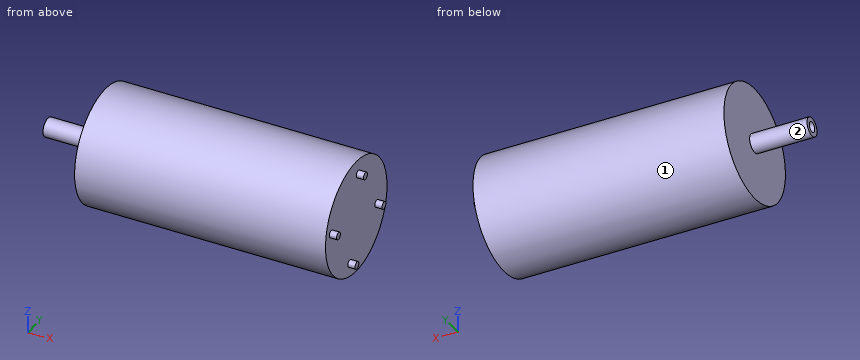
```python
from build123d import *

# Parameters (mm, degrees)
F0_W     = 40
F0_H     = 3
F2_R     = 2.5
F3_DEPTH = 5


with BuildPart() as f1:
    # F0 (on Front) → F1 (revolve)
    with BuildSketch(Plane.XZ):
        with Locations((-34.818123, 5)):
            Rectangle(F0_W, F0_H)
        Polygon((-14.818123, 3.5), (-14.818123, 0), (160.181877, 0), (160.181877, 40), (-14.818123, 40), (-14.818123, 6.5), align=None)
    revolve(axis=Axis((18.749876, 0, 0), (1, 0, 0)))

    # F2 (on face) → F3 (join)
    with BuildSketch(Plane.YZ.offset(160.181877)):
        with Locations((2.648871, 29.522968)):
            Circle(F2_R)
        with Locations((-8.448871, -29.522968)):
            Circle(F2_R)
        with Locations((26.622968, -5.548871)):
            Circle(F2_R)
        with Locations((-32.422968, 5.548871)):
            Circle(F2_R)
    extrude(amount=F3_DEPTH)


solid = f1.part
```
Work out the finished part from the listing and answer in its coordinate system (mm). Face numbers are marked on the shaded views. A direction names the side the tool comes from. Give positions to 0.01 mm unless a question says otherwise; leave off trailing zeros. Order: outer loops, then holes, each group sorted by start corner. A loop starts at its lowest first (then second) coordinate and runs counter-clockwise, first axis right, second up.
1. Section D-D, the plane z = -20 is taken. Determine the outline of the cut face in (x, y).
Result sheet:
outline: (-14.82, -34.64) - (160.18, -34.64) - (160.18, 34.64) - (-14.82, 34.64) - close
2. Section A-A, the plane z = 0 is taken. Determine the outline of the cut face in (x, y), and give its area (3 significant figures).
Result sheet:
outline: (-54.82, -6.5) - (-14.82, -6.5) - (-14.82, -40) - (160.18, -40) - (160.18, 40) - (-14.82, 40) - (-14.82, 6.5) - (-54.82, 6.5) - (-54.82, 3.5) - (-14.82, 3.5) - (-14.82, -3.5) - (-54.82, -3.5) - close
area: 14,200 mm2
3. For the marked faces 1 and 2, determine the directions among +Z, -Z, +X, -X, +Y, -Y from which every point of the face is accessible in a straight line to the end or side of a thin tool.
Result sheet:
face 1: +X, -X
face 2: -X
4. Section B-B, the plane x = -27.5 is taken. Determine the outline of the cut face in (y, z), and give its area (3 significant figures).
Result sheet:
outline: circle Ø13 at (0, 0); hole circle Ø7 at (0, 0)
area: 94.2 mm2
5. Each of these flat-tipped pins is pushed along its axis until it touches: P1, Ø8, axis at y = -23.5, z = 6, coming from the -X side; P2, Ø12, axis at y = 27, z = 27, coming from the +X side; P3, Ø1, axis at x = 20, y = 16, coming from the -Z side. Where does it stop, or does it pass through?
Result sheet:
P1: stops at x = -14.82
P2: stops at x = 160.18
P3: stops at z = -36.87
6. Section C-C, the plane x = 121 is taken. Determine the outline of the cut face in (y, z), and give its area (3 significant figures).
Result sheet:
outline: circle Ø80 at (0, 0)
area: 5,030 mm2
7. Straight lines are drawn through the part: L1, parallel to Z at x = -39.5, y = 0; L2, parallel to X at y = -3.5, z = -15.5. For each, find the intervals that lie inside material, in ascending order.
Result sheet:
L1: z = -6.5 to -3.5, 3.5 to 6.5
L2: x = -14.82 to 160.18
